Check sheet for the modelled part. Datum: model origin and axes. Units: mm. Face numbers are marked on the shaded views. A direction names the side the tool comes from. Round coordinates to 2 decimals unless told otherwise and drop trailing zeros. Write each loop counter-clockwise with the first axis right and the second up, starting at its lowest first coordinate (ties: lowest second). Pieces come first, ordered by that corner, then holes. Notation, with made-up numbers: (-14, 24.5) -> (8, 24.5) arc R12 cw to (8, 29.5) -> close; hole circle Ø8 at (52, 28.25). An arc over 180 degrees is marked (long way). One line per item, written item: value. Start each with the question number.
```python
from build123d import *

# Parameters (mm, degrees)
CONNECTOR_M5X0_8_TAPPED_HOLE_D        = 4.2
SET_SCREW_1_M3X0_5_TAPPED_HOLE_REACH  = 16.681
SET_SCREW_1_M3X0_5_TAPPED_HOLE_BORE_R = 1.25
SET_SCREW_2_PATTERN_COUNT             = 2
EDGE_CHAMFERS_SIZE                    = 0.25


with BuildPart() as part:
    # Body Sketch → Body Revolve (revolve)
    with BuildSketch(Plane(origin=(0, 0, 0), x_dir=(-1, 0, 0), z_dir=(0, 1, 0))):
        Polygon((1, 10.5), (3.7, 10.5), (3.7, 5.5), (5.4, 4), (5.4, 0), (2.5, 0), (2.5, 5), (1, 5), align=None)
    revolve(axis=Axis((0, 0, 0), (0, 0, 1)))

    # Connector M5x0.8 Tapped Hole (through all)
    with Locations(Plane.XY.offset(10.5)):
        with Locations((0, 0)):
            Hole(CONNECTOR_M5X0_8_TAPPED_HOLE_D / 2)

    # Set Screw 1 M3x0.5 Tapped Hole bore (on position points) → Set Screw 1 M3x0.5 Tapped Hole (cut, up to next)
    with BuildSketch(Plane(origin=(5.4, 0, 2.15), x_dir=(0, 1, 0), z_dir=(1, 0, 0)), mode=Mode.PRIVATE) as set_screw_1_m3x0_5_tapped_hole_sk1:
        Circle(SET_SCREW_1_M3X0_5_TAPPED_HOLE_BORE_R)
    set_screw_1_m3x0_5_tapped_hole_tool1 = extrude(set_screw_1_m3x0_5_tapped_hole_sk1.sketch, amount=-SET_SCREW_1_M3X0_5_TAPPED_HOLE_REACH, mode=Mode.PRIVATE) & part.part
    set_screw_1_m3x0_5_tapped_hole = set_screw_1_m3x0_5_tapped_hole_tool1.solids().sort_by_distance((5.4, 0, 2.15))[0]
    add(set_screw_1_m3x0_5_tapped_hole, mode=Mode.SUBTRACT)

    # Set Screw 2 Pattern: Set Screw 1 M3x0.5 Tapped Hole ×2 about axis
    set_screw_2_pattern_axis = Axis((0, 0, 0), (0, 0, 1))
    for i in range(1, SET_SCREW_2_PATTERN_COUNT):
        add(set_screw_1_m3x0_5_tapped_hole.rotate(set_screw_2_pattern_axis, i * 360 / SET_SCREW_2_PATTERN_COUNT), mode=Mode.SUBTRACT)

    # Edge Chamfers
    edge_chamfers_edges = [part.edges().sort_by_distance(p)[0] for p in [
        (5.4, 0, 0),
        (3.7, 0, 10.5),
    ]]
    chamfer(edge_chamfers_edges, length=EDGE_CHAMFERS_SIZE)


solid = part.part
```
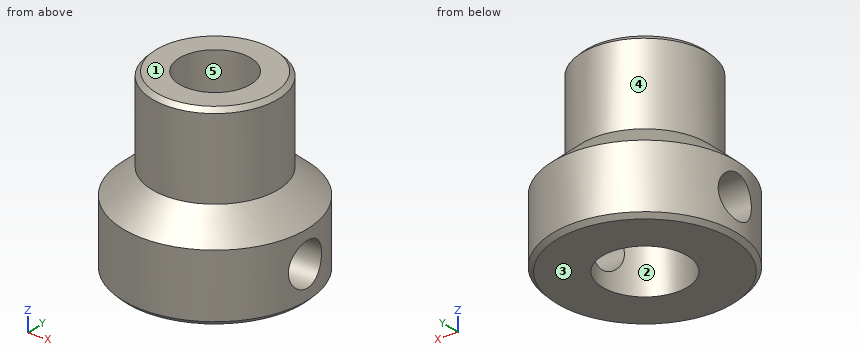
1. Cross-section at A-A (x = 0). Record the cut outline in (y, z).
2. Depth check by flat-ended pin: pin 1 Ø3 at (y, z) = (2.5, 9) entering from -X; pin 2 Ø5 at (x, z) = (-2.5, 7) entering from -Y; pin 3 Ø3 at (x, z) = (-2, 4.5) entering from -Y. Enter the tip coordinate at first touch or a pass-through.
3. Cross-section at B-B (y = 0). Record the cut outline in (x, z).
4. Access from +Z, -Z, +X, -X, +Y, -Y to the whole of each face (thin tool, end or side, straight path). Record for the marked faces 1 and 2.
5. Cross-section at C-C (z = 2.15). Record the cut outline in (x, y), plus the area to 3 significant figures.
6. Cross-section at D-D (z = 4.25). Record the cut outline in (x, y).
7. Material ranges on probe 1 along Y at (x, z) = (0, 6.2); probe 2 along X at (y, z) = (0, 3.5); probe 3 along Y at (x, z) = (-1.75, 7.75), recorded low to high.
8. Release check for a two-part mould opening along Y. For the marked faces 3, 4 and 5 record: +Y half, -Y half, draft (parallel to the pull), parting line (faces both ways), or undercut.
Working result:
1. outline: (-5.4, 0.25) -> (-5.15, 0) -> (-2.5, 0) -> (-2.5, 5) -> (-2.1, 5) -> (-2.1, 10.5) -> (-3.45, 10.5) -> (-3.7, 10.25) -> (-3.7, 5.5) -> (-5.4, 4) -> close; (2.1, 5) -> (2.5, 5) -> (2.5, 0) -> (5.15, 0) -> (5.4, 0.25) -> (5.4, 4) -> (3.7, 5.5) -> (3.7, 10.25) -> (3.45, 10.5) -> (2.1, 10.5) -> close
2. pin 1: stops at x = -3.56
2. pin 2: stops at y = -4.37
2. pin 3: stops at y = -5.37
3. outline: (-5.4, 0.25) -> (-5.15, 0) -> (-2.5, 0) -> (-2.5, 0.9) -> (-5.4, 0.9) -> close; (-5.4, 3.4) -> (-2.5, 3.4) -> (-2.5, 5) -> (-2.1, 5) -> (-2.1, 10.5) -> (-3.45, 10.5) -> (-3.7, 10.25) -> (-3.7, 5.5) -> (-5.4, 4) -> close; (2.1, 5) -> (2.5, 5) -> (2.5, 3.4) -> (5.4, 3.4) -> (5.4, 4) -> (3.7, 5.5) -> (3.7, 10.25) -> (3.45, 10.5) -> (2.1, 10.5) -> close; (2.5, 0) -> (5.15, 0) -> (5.4, 0.25) -> (5.4, 0.9) -> (2.5, 0.9) -> close
4. face 1: +Z, +X, -X, +Y, -Y
4. face 2: -Z
5. outline: (-5.25, -1.25) arc R5.4 ccw to (5.25, -1.25) -> (2.17, -1.25) arc R2.5 cw to (-2.17, -1.25) -> close; (-5.25, 1.25) -> (-2.17, 1.25) arc R2.5 cw to (2.17, 1.25) -> (5.25, 1.25) arc R5.4 ccw to start
5. area: 57.2 mm^2
6. outline: circle Ø10.23 at (0, 0); hole circle Ø5 at (0, 0)
7. probe 1: y = -3.7 to -2.1, 2.1 to 3.7
7. probe 2: x = -5.4 to -2.5, 2.5 to 5.4
7. probe 3: y = -3.26 to -1.16, 1.16 to 3.26
8. face 3: draft
8. face 4: parting line
8. face 5: undercut
